Geometry check sheet. Reference: the model listing, model coordinates, mm. Face numbers are marked on the shaded views. A direction names the side the tool comes from. Coordinates: 2 decimals unless noted, no trailing zeros. Write each loop counter-clockwise with the first axis right and the second up, starting at its lowest first coordinate (ties: lowest second). Pieces come first, ordered by that corner, then holes. Notation, with made-up numbers: (12, 34) -> (70, 34) arc R21 ccw to (70, 52) -> close; hole circle Ø6 at (-4.5, 24). An arc over 180 degrees is marked (long way). Answer in a Markdown table with one row per item. Add a question column.
1. Scan lines: L1, parallel to Z at x = 2.5, y = 1; L2, parallel to Y at x = 3, z = -1.5; L3, parallel to X at y = -11, z = 0. Record each from-to range of solid material in increasing order. Write a range as from..to.
2. Depth check by flat-ended pin: P1, Ø10, axis at y = -5.5, z = -9.5, coming from the +X side; P2, Ø1.5, axis at x = 10.5, z = 10.5, coming from the +Y side; P3, Ø1.4, axis at x = 4, z = -1, coming from the +Y side; P4, Ø2, axis at x = 10.5, y = -5.5, coming from the +Z side. Enter the tip coordinate at first touch or a pass-through.
3. Cross-section at B-B on x = 7.75. Record the cut outline in (y, z).
4. Set-up check for the marked faces 1, 2 and 3: record each of +Z, -Z, +X, -X, +Y, -Y from which the full face is reachable in a straight line by a thin tool's end or side.
5. Cross-section at A-A on z = 0. Give the number of separate pieces and of enclosed holes in the cut face, and give its area (3 significant figures).
6. Mould release check, pull along Y, two halves, no side actions. Record for the marked faces 4, 5 and 6: pulls with the +Y half, pulls with the -Y half, needs draft (parallel to the pull), parting line crosses it, or undercut.
```python
from build123d import *

# Parameters (mm, degrees)
SKETCH_1_R                      = 12.55
EXTRUDE_1_DEPTH                 = 10
SKETCH_2_R                      = 3
CUT_EXTRUDE_1_DEPTH             = 7
CUT_EXTRUDE_2_REACH             = 22.372
SKETCH_3_R                      = 1
CUT_EXTRUDE_2_DIRECTION_2_REACH = 22.372
CUT_EXTRUDE_3_DEPTH             = 21
CUT_EXTRUDE_3_DEPTH_BACK        = 19
SKETCH_4_R                      = 1
EXTRUDE_2_DEPTH                 = 2.5
EXTRUDE_2_DEPTH_BACK            = 1
SKETCH_5_R                      = 16
SKETCH_6_R                      = 12.6
CUT_EXTRUDE_4_DEPTH             = 2.5
FILLET_1_R                      = 2
SKETCH_7_W                      = 2.5
SKETCH_7_H                      = 10
CUT_EXTRUDE_5_DEPTH             = 21.5
CUT_EXTRUDE_7_DEPTH             = 1.5
SKETCH_13_W                     = 4.62
SKETCH_13_H                     = 1.5
CUT_EXTRUDE_8_DEPTH             = 4
SKETCH_14_W                     = 1.5
SKETCH_14_H                     = 4.62
CUT_EXTRUDE_9_DEPTH             = 4
CUT_EXTRUDE_10_DEPTH            = 1.5


with BuildPart() as part:
    # 草图1 → 凸台-拉伸1 (new body)
    with BuildSketch(Plane(origin=(0, 0, 0), x_dir=(0, 0, -1), z_dir=(1, 0, 0))):
        Circle(SKETCH_1_R)
    extrude(amount=EXTRUDE_1_DEPTH)

    # 草图2 → 切除-拉伸1 (cut)
    with BuildSketch(Plane.ZY):
        Circle(SKETCH_2_R)
    extrude(amount=-CUT_EXTRUDE_1_DEPTH, mode=Mode.SUBTRACT)

    # 草图3 → 切除-拉伸2 (cut, up to next)
    with BuildSketch(Plane(origin=(0, 0, 0), x_dir=(1, 0, 0), z_dir=(0, 1, 0)), mode=Mode.PRIVATE) as cut_extrude_2_sk1:
        with Locations(Location((4, 0, 0), (0, 0, 270))):
            Circle(SKETCH_3_R)
    cut_extrude_2_tool1 = extrude(cut_extrude_2_sk1.sketch, amount=-CUT_EXTRUDE_2_REACH, mode=Mode.PRIVATE) & part.part
    add(cut_extrude_2_tool1.solids().sort_by_distance((4, 0, 0))[0], mode=Mode.SUBTRACT)

    # 草图3 → 切除-拉伸2 direction 2 (cut, up to next)
    with BuildSketch(Plane(origin=(0, 0, 0), x_dir=(1, 0, 0), z_dir=(0, 1, 0)), mode=Mode.PRIVATE) as cut_extrude_2_direction_2_sk1:
        with Locations(Location((4, 0, 0), (0, 0, 270))):
            Circle(SKETCH_3_R)
    cut_extrude_2_direction_2_tool1 = extrude(cut_extrude_2_direction_2_sk1.sketch, amount=CUT_EXTRUDE_2_DIRECTION_2_REACH, mode=Mode.PRIVATE) & part.part
    add(cut_extrude_2_direction_2_tool1.solids().sort_by_distance((4, 0, 0))[0], mode=Mode.SUBTRACT)

    # 草图4 → 切除-拉伸3 (cut, two sides: drawn at the far end of the back side and taken through both)
    with BuildSketch(Plane.XY.offset(-CUT_EXTRUDE_3_DEPTH_BACK)):
        with Locations(Location((4, 0, 0), (0, 0, 180))):
            Circle(SKETCH_4_R)
    extrude(amount=CUT_EXTRUDE_3_DEPTH + CUT_EXTRUDE_3_DEPTH_BACK, mode=Mode.SUBTRACT)

    # 草图5 → 凸台-拉伸2 (add, two sides: drawn at the far end of the back side and taken through both)
    with BuildSketch(Plane(origin=(10, 0, 0), x_dir=(0, 0, -1), z_dir=(1, 0, 0)).offset(-EXTRUDE_2_DEPTH_BACK)):
        Circle(SKETCH_5_R)
    extrude(amount=EXTRUDE_2_DEPTH + EXTRUDE_2_DEPTH_BACK)

    # 草图6 → 切除-拉伸4 (cut)
    with BuildSketch(Plane(origin=(12.5, 0, 0), x_dir=(0, 0, -1), z_dir=(1, 0, 0))):
        Circle(SKETCH_6_R)
    extrude(amount=-CUT_EXTRUDE_4_DEPTH, mode=Mode.SUBTRACT)

    # 圆角1
    fillet_1_edges = [part.edges().sort_by_distance(p)[0] for p in [
        (9, 0, 12.55),
    ]]
    fillet(fillet_1_edges, radius=FILLET_1_R)

    # 草图7 → 切除-拉伸5 (cut)
    with BuildSketch(Plane.XY):
        with Locations((11.25, 0)):
            Rectangle(SKETCH_7_W, SKETCH_7_H)
    extrude(amount=-CUT_EXTRUDE_5_DEPTH, mode=Mode.SUBTRACT)

    # 草图11 → 切除-拉伸7 (cut)
    with BuildSketch(Plane(origin=(0, 6, 0), x_dir=(1, 0, 0), z_dir=(0, 1, 0))):
        Polygon((4, 2.309401077), (2, 1.154700538), (2, -1.154700538), (4, -2.309401077), (6, -1.154700538), (6, 1.154700538), align=None)
    cut_extrude_7 = extrude(amount=CUT_EXTRUDE_7_DEPTH, mode=Mode.SUBTRACT)

    # 草图13 → 切除-拉伸8 (cut)
    with BuildSketch(Plane.ZY):
        with Locations((0, 6.75)):
            Rectangle(SKETCH_13_W, SKETCH_13_H)
    cut_extrude_8 = extrude(amount=-CUT_EXTRUDE_8_DEPTH, mode=Mode.SUBTRACT)

    # 草图14 → 切除-拉伸9 (cut)
    with BuildSketch(Plane.ZY):
        with Locations((6.75, 0)):
            Rectangle(SKETCH_14_W, SKETCH_14_H)
    cut_extrude_9 = extrude(amount=-CUT_EXTRUDE_9_DEPTH, mode=Mode.SUBTRACT)

    # 草图9 → 切除-拉伸10 (cut)
    with BuildSketch(Plane.XY.offset(6)):
        Polygon((4, 2.309401077), (2, 1.154700538), (2, -1.154700538), (4, -2.309401077), (6, -1.154700538), (6, 1.154700538), align=None)
    cut_extrude_10 = extrude(amount=CUT_EXTRUDE_10_DEPTH, mode=Mode.SUBTRACT)

    # 镜向1: 切除-拉伸9, 切除-拉伸10 across plane
    add(cut_extrude_9.mirror(Plane.XY), mode=Mode.SUBTRACT)
    add(cut_extrude_10.mirror(Plane.XY), mode=Mode.SUBTRACT)

    # 镜向2: 切除-拉伸7, 切除-拉伸8 across plane
    add(cut_extrude_7.mirror(Plane.ZX), mode=Mode.SUBTRACT)
    add(cut_extrude_8.mirror(Plane.ZX), mode=Mode.SUBTRACT)


solid = part.part
```
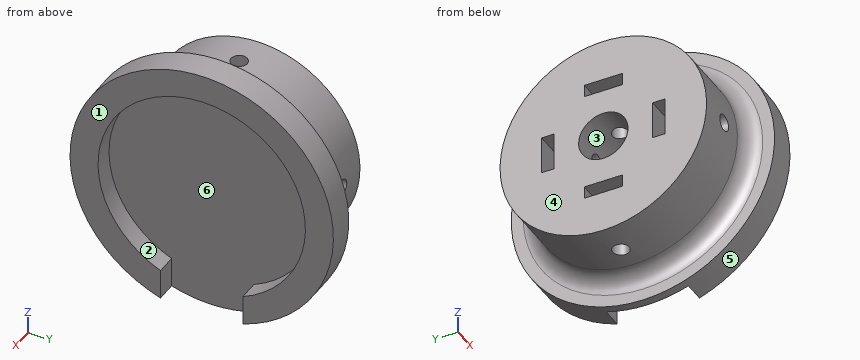
Results found:
| question | item | result |
|---|---|---|
| 1 | L1 | z = -12.51..-7.5, -6..-2.83, 2.83..6, 7.5..12.51 |
| 1 | L2 | y = -12.46..-7.5, -6..-2.6, 2.6..6, 7.5..12.46 |
| 1 | L3 | x = 0..3, 5..10 |
| 2 | P1 | stops at x = 12.5 |
| 2 | P2 | stops at y = 12.69 |
| 2 | P3 | stops at y = 12.53 |
| 2 | P4 | stops at z = 15.35 |
| 3 | outline | circle Ø25.39 at (0, 0) |
| 4 | face 1 | +Z, -Z, +X, +Y, -Y |
| 4 | face 2 | +X |
| 4 | face 3 | -X |
| 5 | separate pieces | 5 |
| 5 | enclosed holes | 0 |
| 5 | area | 184 mm^2 |
| 6 | face 4 | needs draft |
| 6 | face 5 | parting line crosses it |
| 6 | face 6 | undercut |
